```python
from build123d import *

# Parameters (mm, degrees)
BOSS_EXTRUDE1_START = -11
SKETCH2_R           = 5
BOSS_EXTRUDE1_DEPTH = 3
FILLET1_R           = 5


with BuildPart() as part:
    # Sketch1 → Revolve1 (revolve)
    with BuildSketch(Plane.XY, mode=Mode.PRIVATE) as revolve1_sk:
        with BuildLine():
            Line((-16.8, 4), (-19, 4))
            Line((-19, 4), (-19, 0))
            Line((-19, 0), (-7, 0))
            Line((-7, 0), (-7, 4))
            Line((-7, 4), (-12.2, 4))
            ThreePointArc((-12.2, 4), (-14.5, 2.757481343), (-16.8, 4))
        make_face()
    revolve(revolve1_sk.sketch.rotate(Axis((0, 8.369163349, 0), (0, -1, 0)), 270), axis=Axis((0, 8.369163349, 0), (0, -1, 0)))

    # Sketch2 → Boss-Extrude1 (add)
    with BuildSketch(Plane(origin=(0, 0, 0), x_dir=(0, 0, -1), z_dir=(1, 0, 0)).offset(BOSS_EXTRUDE1_START)):
        with BuildLine():
            Line((13, 0), (-13, 0))
            add(Edge.make_bspline(
                [(-5.875693444, -36.071419141), (-11.248074258, -24.550311306), (-13, -12.25607796), (-13, 0)],
                knots=[0, 0, 0, 0, 1, 1, 1, 1], degree=3))
            ThreePointArc((-5.875693444, -36.071419141), (10.071419141, -41.875693444), (15.875693444, -25.928580859))
            add(Edge.make_bspline(
                [(15.875693444, -25.928580859), (12.156143996, -17.951981325), (13, -8.695854173), (13, 0)],
                knots=[0, 0, 0, 0, 1, 1, 1, 1], degree=3))
        make_face()
        with Locations((5, -31)):
            Circle(SKETCH2_R, mode=Mode.SUBTRACT)
    boss_extrude1 = extrude(amount=-BOSS_EXTRUDE1_DEPTH)

    # Mirror1: Boss-Extrude1 across plane
    add(boss_extrude1.mirror(Plane(origin=(0, 0, 0), x_dir=(0, 0, 1), z_dir=(1, 0, 0))))

    # Fillet1
    fillet1_edges = [part.edges().sort_by_distance(p)[0] for p in [
        (0, 4, -16.8),
    ]]
    fillet(fillet1_edges, radius=FILLET1_R)


solid = part.part
```
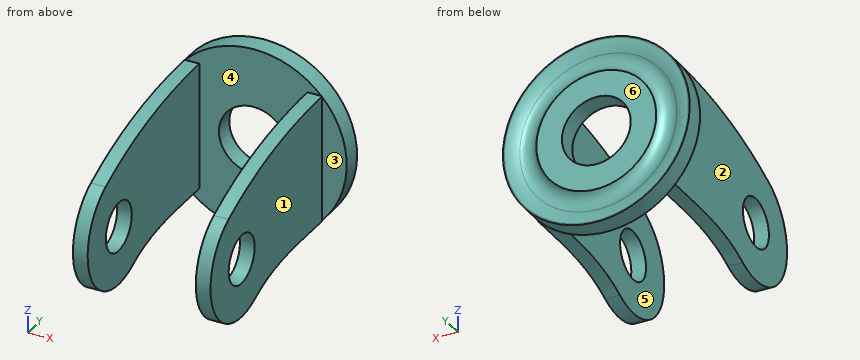
Geometry check sheet. Reference: the model listing, model coordinates, mm. Face numbers are marked on the shaded views. A direction names the side the tool comes from. Give positions to 0.01 mm unless a question says otherwise; leave off trailing zeros.
1) Release check for a two-part mould opening along X. For the marked faces 1, 2, 3 and 4 record: pulls with the +X half, pulls with the -X half, needs draft (parallel to the pull), parting line crosses it, or undercut.
2) Gauge pin test, flat ends, axial feed: pin 1 (4 mm diameter, centred on x = 4.5, z = -2.5, fed in from -Y); pin 2 (11.5 mm diameter, centred on y = -31, z = -5, fed in from +X); pin 3 (1.5 mm diameter, centred on y = -18, z = 8.5, fed in from -X). Record the tip position at first contact, or that the pin passes through.
3) Section check A-A, the plane z = -5. State how many separate pieces and enclosed holes the cut face has, and give its area (3 significant figures).
4) Material ranges on L1, parallel to X at y = 1.5, z = 0; L2, parallel to X at y = -3, z = 7; L3, parallel to Y at x = 4, z = -11, recorded low to high.
5) Access from +Z, -Z, +X, -X, +Y, -Y to the whole of each face (thin tool, end or side, straight path). Record for the marked faces 5 and 6.
Computed:
1. face 1: pulls with the +X half
1. face 2: pulls with the -X half
1. face 3: needs draft
1. face 4: undercut
2. pin 1: stops at y = 0
2. pin 2: stops at x = 14
2. pin 3: stops at x = -14
3. separate pieces: 4
3. enclosed holes: 0
3. area: 296 mm2
4. L1: x = -19 to -7, 7 to 19
4. L2: x = -14 to -11, 11 to 14
4. L3: y = 0 to 4
5. face 5: +Z, -Z, -Y
5. face 6: +Z, -Z, +X, -X, +Y
